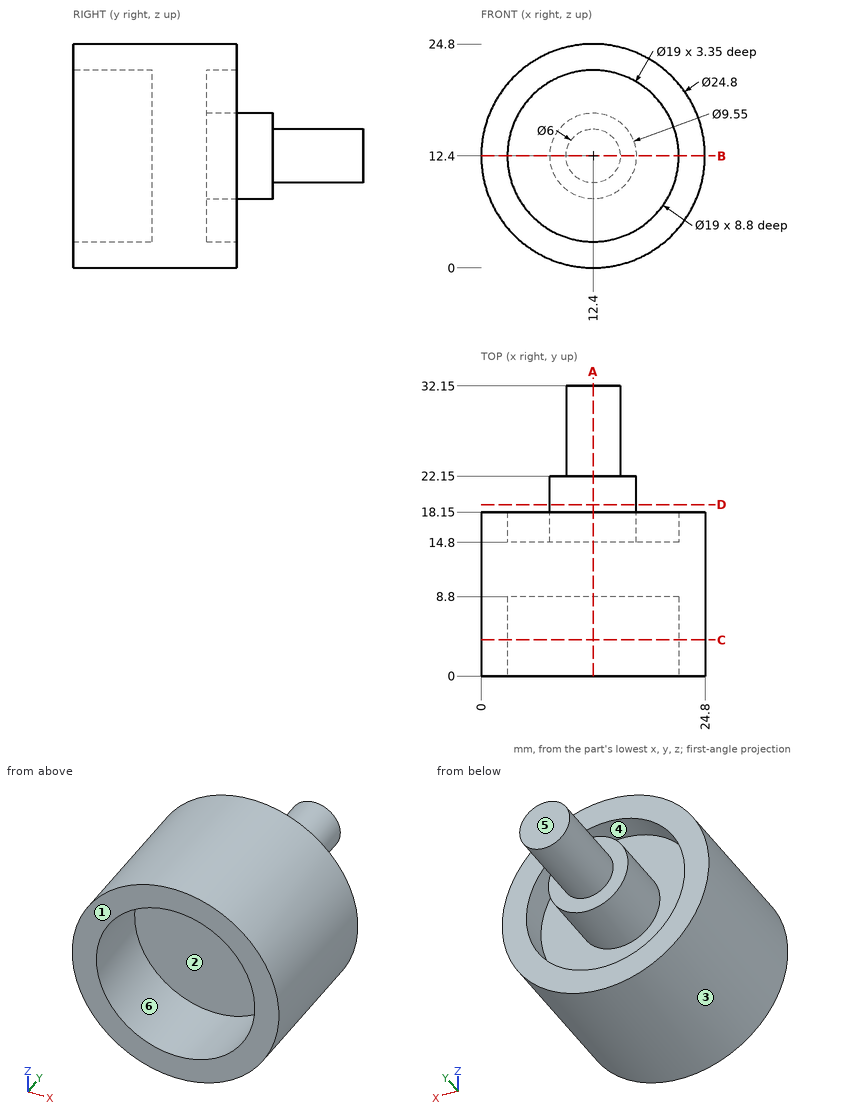
Here's the drawing with two shaded views (mm, measured from the low corner). I have some questions. A direction names the side the tool comes from. Coordinates: 2 decimals unless noted, no trailing zeros. Loops run counter-clockwise (first coordinate to the right, second up) from the corner with the lowest first, then second, coordinate; pieces in that order, holes last. Notation, with made-up numbers: (1.5, -38) -> (50.5, -38) arc R20 cw to (50.5, -12) -> close; hole circle Ø11 at (19, 81). An arc over 180 degrees is marked (long way). Put each result on its own line as item: value. Start each with the question number.
Q1. I want a section at D-D (y = 19). Write out the boundary of the cut face in (x, z) (3 decimals).
Q2. I want a section at C-C (y = 4). Write out the boundary of the cut face in (x, z).
Q3. I want a section at B-B (z = 12.4). Write out the boundary of the cut face in (x, y) (3 decimals).
Q4. I'm going to push flat-ended pins straight in: P1, Ø6, axis at x = 4.5, z = 21, coming from the +Y side; P2, Ø11.5, axis at x = 12.4, z = 12.4, coming from the -Y side; P3, Ø1.5, axis at y = 19.5, z = 10.5, coming from the -X side. Where does each tip first touch, or does it pass through?
Q5. Thinking about a two-plate mould opening in X: for the marked faces 1, 2 and 3, which applies, pulls with the +X half, pulls with the -X half, needs draft (parallel to the pull), parting line crosses it, or undercut?
Q6. If I drill on line 1 (X direction, y = 15.5, z = 12.4) (3 decimals); line 2 (X direction, y = 2.75, z = 12.4); line 3 (Z direction, x = 10, y = 18), over which ranges is the centre line in solid material (lowest first)? Write a range as [from, to].
Q7. I want a section at A-A (x = 12.4). Write out the boundary of the cut face in (y, z) (3 decimals), plus the area to 3 significant figures.
Q8. For the marked faces 4, 5 and 6, which set-ups out of +Z, -Z, +X, -X, +Y, -Y let a thin tool reach every point of the face, with its end or its side?
Taken from the geometry:
1. outline: circle Ø9.55 at (12.4, 12.4)
2. outline: circle Ø24.8 at (12.4, 12.4); hole circle Ø19 at (12.4, 12.4)
3. outline: (0, 0) -> (2.9, 0) -> (2.9, 8.8) -> (21.9, 8.8) -> (21.9, 0) -> (24.8, 0) -> (24.8, 18.15) -> (21.9, 18.15) -> (21.9, 14.8) -> (17.175, 14.8) -> (17.175, 22.15) -> (15.4, 22.15) -> (15.4, 32.15) -> (9.4, 32.15) -> (9.4, 22.15) -> (7.625, 22.15) -> (7.625, 14.8) -> (2.9, 14.8) -> (2.9, 18.15) -> (0, 18.15) -> close
4. P1: stops at y = 18.15
4. P2: stops at y = 8.8
4. P3: stops at x = 7.77
5. face 1: needs draft
5. face 2: undercut
5. face 3: parting line crosses it
6. line 1: x = [0, 2.9], [7.625, 17.175], [21.9, 24.8]
6. line 2: x = [0, 2.9], [21.9, 24.8]
6. line 3: z = [0.23, 3.21], [8.27, 16.53], [21.59, 24.57]
7. outline: (0, 0) -> (18.15, 0) -> (18.15, 2.9) -> (14.8, 2.9) -> (14.8, 7.625) -> (22.15, 7.625) -> (22.15, 9.4) -> (32.15, 9.4) -> (32.15, 15.4) -> (22.15, 15.4) -> (22.15, 17.175) -> (14.8, 17.175) -> (14.8, 21.9) -> (18.15, 21.9) -> (18.15, 24.8) -> (0, 24.8) -> (0, 21.9) -> (8.8, 21.9) -> (8.8, 2.9) -> (0, 2.9) -> close
7. area: 349 mm2
8. face 4: +Y
8. face 5: +Z, -Z, +X, -X, +Y
8. face 6: -Y
